Design review of the part built by this model. Coordinates are the model's own, in mm. Face numbers are marked on the shaded views. A direction names the side the tool comes from. Give positions to 0.01 mm unless a question says otherwise; leave off trailing zeros. Loops run counter-clockwise (first coordinate to the right, second up) from the corner with the lowest first, then second, coordinate; pieces in that order, holes last. Notation, with made-up numbers: (43, 37) - (78, 37) arc R33 ccw to (78, 74) - close; hole circle Ø6 at (19.25, 62.25). An arc over 180 degrees is marked (long way). Write each question's results on one line, items separated by ' | '.
from build123d import *

# Parameters (mm, degrees)
ESQUISSE1_W        = 120
ESQUISSE1_H        = 55
ESQUISSE1_R        = 1.6
BOSS_EXTRU_1_DEPTH = 1.6
ESQUISSE2_W        = 43.050312428
ESQUISSE2_H        = 37.603564561
ESQUISSE2_W_2      = 6.539195339
ESQUISSE2_H_2      = 27.81484763
BOSS_EXTRU_2_DEPTH = 18


with BuildPart() as part:
    # Esquisse1 → Boss.-Extru.1 (new body)
    with BuildSketch(Plane.XY):
        Rectangle(ESQUISSE1_W, ESQUISSE1_H)
        with Locations((-56.5, 24)):
            Circle(ESQUISSE1_R, mode=Mode.SUBTRACT)
        with Locations((56.5, 24)):
            Circle(ESQUISSE1_R, mode=Mode.SUBTRACT)
        with Locations((56.5, -24)):
            Circle(ESQUISSE1_R, mode=Mode.SUBTRACT)
        with Locations((-56.5, -24)):
            Circle(ESQUISSE1_R, mode=Mode.SUBTRACT)
    extrude(amount=BOSS_EXTRU_1_DEPTH)

    # Esquisse2 → Boss.-Extru.2 (add)
    with BuildSketch(Plane.XY.offset(1.6)):
        with Locations((-29.757687253, 0.675058423)):
            Rectangle(ESQUISSE2_W, ESQUISSE2_H)
        with Locations((55.030096994, 2.76225902)):
            Rectangle(ESQUISSE2_W_2, ESQUISSE2_H_2)
    extrude(amount=BOSS_EXTRU_2_DEPTH)


solid = part.part
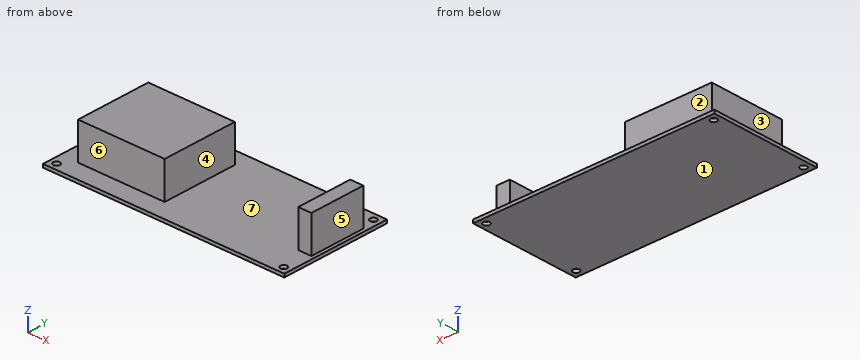
(1) Wall thickness on line 1 along Y through (x, z) = (-56.5, 0.65); line 2 along X through (y, z) = (9.5, 4); line 3 along Z through (x, y) = (-13, 21): over which ranges is each line inside the solid? List them lowest first. Write a range as from..to.
Answers below:
line 1: -27.5..-25.6, -22.4..22.4, 25.6..27.5 | line 2: -51.28..-8.23, 51.76..58.3 | line 3: 0..1.6
(2) Take a section at D-D on y = -9. Give the boundary of the cut face in (x, z), plus the area to 3 significant figures.
Answers below:
outline: (-60, 0) - (60, 0) - (60, 1.6) - (58.3, 1.6) - (58.3, 19.6) - (51.76, 19.6) - (51.76, 1.6) - (-8.23, 1.6) - (-8.23, 19.6) - (-51.28, 19.6) - (-51.28, 1.6) - (-60, 1.6) - close | area: 1,080 mm2
(3) Take a section at C-C on z = 11.5. Give the boundary of the cut face in (x, y), plus the area to 3 significant figures.
Answers below:
outline: (-51.28, -18.13) - (-8.23, -18.13) - (-8.23, 19.48) - (-51.28, 19.48) - close; (51.76, -11.15) - (58.3, -11.15) - (58.3, 16.67) - (51.76, 16.67) - close | area: 1,800 mm2
(4) Take a section at B-B on y = 24. Give the boundary of the cut face in (x, z).
Answers below:
outline: (-60, 0) - (-58.1, 0) - (-58.1, 1.6) - (-60, 1.6) - close; (-54.9, 0) - (54.9, 0) - (54.9, 1.6) - (-54.9, 1.6) - close; (58.1, 0) - (60, 0) - (60, 1.6) - (58.1, 1.6) - close
(5) Tool access review of the marked faces 1, 2 and 3: name each direction out of +Z, -Z, +X, -X, +Y, -Y from which nothing blocks a thin tool from reaching the whole face with its end or side.
Answers below:
face 1: -Z, +X, -X, +Y, -Y | face 2: +Z, +X, -X, +Y | face 3: +Z, -X, +Y, -Y
(6) Insertion check: P1, Ø2.5, axis at x = -56.5, y = 24, coming from the -Z side; P2, Ø4, axis at y = 14, z = 15.5, coming from the -X side; P3, Ø9, axis at y = 1, z = 10, coming from the +X side; P4, Ø7, axis at x = 54, z = 12.5, coming from the +Y side. Each pin has a flat end and moves straight along its axis. Give the tip position at first contact, or say it passes through.
Answers below:
P1: through | P2: x = -51.28 | P3: x = 58.3 | P4: y = 16.67
(7) Draft analysis for pull direction X (two halves, no side actions). For the marked faces 4, 5, 6 and 7, state which applies: pulls with the +X half, pulls with the -X half, needs draft (parallel to the pull), parting line crosses it, or undercut.
Answers below:
face 4: undercut | face 5: pulls with the +X half | face 6: needs draft | face 7: undercut
(8) Take a section at A-A on x = -56.5. Give the boundary of the cut face in (y, z).
Answers below:
outline: (-27.5, 0) - (-25.6, 0) - (-25.6, 1.6) - (-27.5, 1.6) - close; (-22.4, 0) - (22.4, 0) - (22.4, 1.6) - (-22.4, 1.6) - close; (25.6, 0) - (27.5, 0) - (27.5, 1.6) - (25.6, 1.6) - close
